Geometry check sheet. Reference: the model listing, model coordinates, mm. Face numbers are marked on the shaded views. A direction names the side the tool comes from. Round coordinates to 2 decimals unless told otherwise and drop trailing zeros. Order: outer loops, then holes, each group sorted by start corner. A loop starts at its lowest first (then second) coordinate and runs counter-clockwise, first axis right, second up.
(1) Draft check along Y on the marked faces 4, 5 and 6. Enter one of: pulls with the +Y half, pulls with the -Y half, needs draft (parallel to the pull), parting line crosses it, or undercut.
(2) Cross-section at A-A on x = 117.5. Enter the section's corners in (y, z).
(3) Thickness scan on L1, parallel to X at y = 0, z = 26; L2, parallel to Y at x = 58, z = 0; L3, parallel to X at y = -18, z = 0. Record the ranges inside material, lowest first.
(4) Cross-section at B-B on x = 33. Enter the section's corners in (y, z).
(5) Gauge pin test, flat ends, axial feed: P1, Ø8, axis at x = 25, z = 0, coming from the +Y side; P2, Ø5.5, axis at x = 89.5, y = 28, coming from the -Z side; P3, Ø2, axis at x = 109.5, z = 4, coming from the -Y side; P4, Ø3, axis at x = 50, y = 19.5, coming from the -Z side. Record the tip position at first contact, or that the pin passes through.
(6) Set-up check for the marked faces 1, 2 and 3: record each of +Z, -Z, +X, -X, +Y, -Y from which the full face is reachable in a straight line by a thin tool's end or side.
(7) Cross-section at C-C on x = 62. Enter the section's corners in (y, z).
from build123d import *

# Parameters (mm, degrees)
CUT_EXTRUDE_9_DEPTH         = 191.91883092
CUT_EXTRUDE_9_DEPTH_BACK    = 191.91883092
SKETCH_6_W                  = 50
SKETCH_6_H                  = 5.5
CUT_EXTRUDE_4_DEPTH         = 5
CUT_EXTRUDE_10_DEPTH        = 191.91883092
CUT_EXTRUDE_10_DEPTH_BACK   = 191.91883092
SKETCH_16_R                 = 5
HOLE_WIZARD_0_15_32_1_D     = 32
HOLE_WIZARD_0_15_32_1_DEPTH = 50
HOLE_WIZARD_0_15_32_1_TIP   = 9.613769904
CHAMFER_3_SIZE              = 2
CHAMFER_4_SIZE              = 2.5


with BuildPart() as part:
    # Эскиз1 → Повернуть1 (revolve)
    with BuildSketch(Plane.XY, mode=Mode.PRIVATE) as revolve_1_sk:
        Polygon((0, 16), (0, 20), (55, 20), (55, 30), (135, 30), (135, 45), (180, 45), (180, 16), align=None)
    revolve(revolve_1_sk.sketch.rotate(Axis((0, 0, 0), (-1, 0, 0)), 90), axis=Axis((0, 0, 0), (-1, 0, 0)))

    # Эскиз15 → Вырез-Вытянуть9 (cut, two sides: drawn at the far end of the back side and taken through both)
    with BuildSketch(Plane(origin=(180, 0, 0), x_dir=(0, 0, -1), z_dir=(1, 0, 0)).offset(-CUT_EXTRUDE_9_DEPTH_BACK)):
        with BuildLine():
            Line((-35, -28.284271247), (-35, 28.284271247))
            ThreePointArc((-35, 28.284271247), (-45, 0), (-35, -28.284271247))
        make_face()
    extrude(amount=CUT_EXTRUDE_9_DEPTH + CUT_EXTRUDE_9_DEPTH_BACK, mode=Mode.SUBTRACT)

    # Эскиз6 → Вырез-Вытянуть4 (cut, symmetric)
    with BuildSketch(Plane.XY):
        with Locations((95, 27.25)):
            Rectangle(SKETCH_6_W, SKETCH_6_H)
    extrude(amount=CUT_EXTRUDE_4_DEPTH, both=True, mode=Mode.SUBTRACT)

    # Эскиз16 → Вырез-Вытянуть10 (cut, two sides: drawn at the far end of the back side and taken through both)
    with BuildSketch(Plane(origin=(0, 0, 0), x_dir=(1, 0, 0), z_dir=(0, 1, 0)).offset(-CUT_EXTRUDE_10_DEPTH_BACK)):
        with Locations(Location((25, 0, 0), (0, 0, 270))):
            Circle(SKETCH_16_R)
    extrude(amount=CUT_EXTRUDE_10_DEPTH + CUT_EXTRUDE_10_DEPTH_BACK, mode=Mode.SUBTRACT)

    # Диаметр отверстия Ø0.15 (32)1
    with Locations(Plane.XY.offset(35)):
        with Locations((157.5, 0)):
            Hole(HOLE_WIZARD_0_15_32_1_D / 2, depth=HOLE_WIZARD_0_15_32_1_DEPTH)
            with Locations((0, 0, -(HOLE_WIZARD_0_15_32_1_DEPTH + HOLE_WIZARD_0_15_32_1_TIP / 2))):  # 118° drill point
                Cone(0, HOLE_WIZARD_0_15_32_1_D / 2, HOLE_WIZARD_0_15_32_1_TIP, mode=Mode.SUBTRACT)

    # Фаска3
    chamfer_3_edges = [part.edges().sort_by_distance(p)[0] for p in [
        (55, 0, 30),
        (0, 0, 20),
    ]]
    chamfer(chamfer_3_edges, length=CHAMFER_3_SIZE)

    # Фаска4
    chamfer_4_edges = [part.edges().sort_by_distance(p)[0] for p in [
        (180, 0, -45),
        (135, 0, -45),
    ]]
    chamfer(chamfer_4_edges, length=CHAMFER_4_SIZE)


solid = part.part
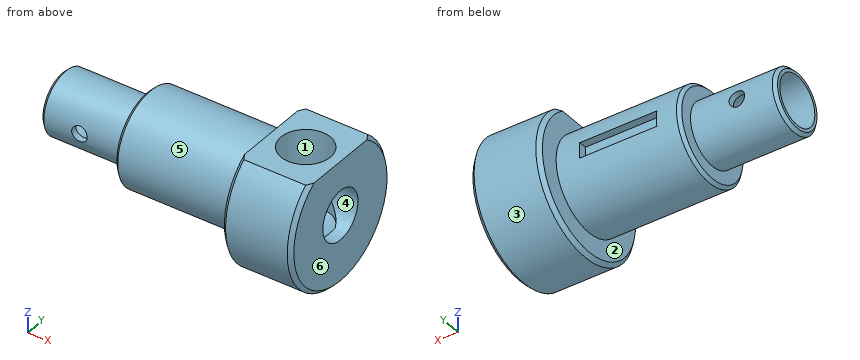
Found:
1. face 4: undercut
1. face 5: parting line crosses it
1. face 6: needs draft
2. outline: (24.5, -5) - (24.5, 5) - (29.58, 5) arc R30 ccw (long way) to (29.58, -5) - close; hole circle Ø32 at (0, 0)
3. L1: x = 55 to 141.5, 173.5 to 180
3. L2: y = -30 to -16, 16 to 30
3. L3: x = 0 to 20, 30 to 180
4. outline: circle Ø40 at (0, 0); hole circle Ø32 at (0, 0)
5. P1: passes through
5. P2: stops at z = -16.2
5. P3: stops at y = -29.85
5. P4: stops at z = -8.72
6. face 1: +Z
6. face 2: -X
6. face 3: +X, -X
7. outline: circle Ø60 at (0, 0); hole circle Ø32 at (0, 0)
